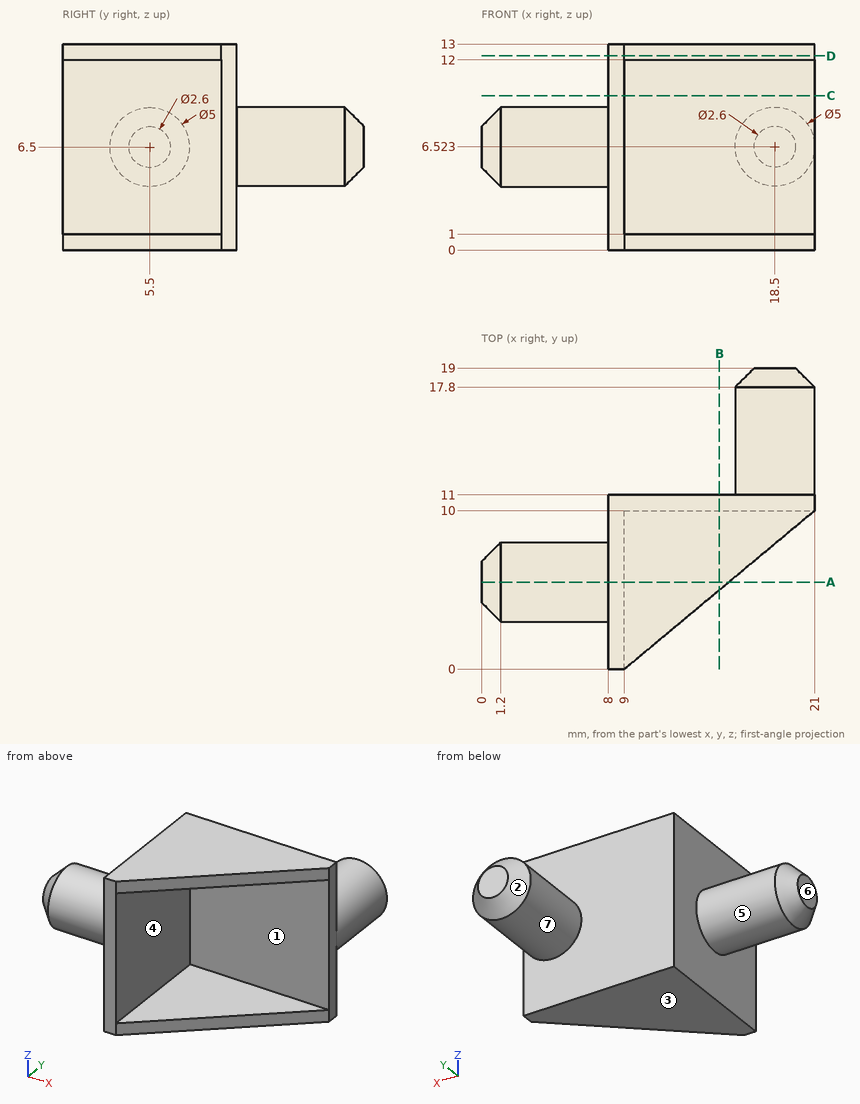
Drawing for the job (mm, zero at the part's lowest x, y, z). A direction names the side the tool comes from. Round coordinates to 2 decimals unless told otherwise and drop trailing zeros. Write each loop counter-clockwise with the first axis right and the second up, starting at its lowest first coordinate (ties: lowest second). Pieces come first, ordered by that corner, then holes. Notation, with made-up numbers: M 3,-27 L 43,-27 A29 ccw 43,-6 Z; hole C 63,29 d9. An arc over 180 degrees is marked long. Answer as a JSON object with one key per item and string values. Group by question number.
(1) Flat gauge pins, fed straight in: pin 1 (4 mm diameter, centred on x = 15, z = 7, fed in from +Y); pin 2 (1 mm diameter, centred on x = 13.5, z = 3, fed in from -Y); pin 3 (4 mm diameter, centred on x = 3, z = 9, fed in from -Y). Where does each tip first touch, or does it go through?
(2) Cut at A-A (y = 5.5). Give the cut face in (x, z).
(3) Which spindle directions (+Z, -Z, +X, -X, +Y, -Y) get a long thin tool onto all of the face, cutting with end or side? Do the marked faces 4, 5, 6 and 7. Say none if no direction does.
(4) Cut at D-D (z = 12.25). Give the cut face in (x, y), and give its area (3 significant figures).
(5) Cut at B-B (x = 15). Give the cut face in (y, z).
(6) Drill centre lines: L1, parallel to Z at x = 10.75, y = 2; L2, parallel to X at y = 10.5, z = 8.75; L3, parallel to Y at x = 13, z = 2. Where is each one in solid material? Low to high.
(7) Cut at C-C (z = 9.75). Give the cut face in (x, y).
(8) Mould opens along Z. For the marked faces 1, 2 and 3 say: pulls with the +Z half, pulls with the -Z half, needs draft (parallel to the pull), parting line crosses it, or undercut.
Responses:
{
 "1": {"pin 1": "stops at y = 18.77", "pin 2": "stops at y = 10", "pin 3": "stops at y = 3.05"},
 "2": {"outline": "M 0,5.2 L 1.2,4 L 8,4 L 8,0 L 15.6,0 L 15.6,1 L 9,1 L 9,12 L 15.6,12 L 15.6,13 L 8,13 L 8,9 L 1.2,9 L 0,7.8 Z"},
 "3": {"face 4": "+X, -Y", "face 5": "-X", "face 6": "+Z, -Z, -X, +Y, -Y", "face 7": "+Y"},
 "4": {"outline": "M 8,0 L 9,0 L 21,10 L 21,11 L 8,11 Z", "area": "83.0 mm2"},
 "5": {"outline": "M 5,0 L 11,0 L 11,13 L 5,13 L 5,12 L 10,12 L 10,1 L 5,1 Z"},
 "6": {"L1": "z = 0 to 1, 12 to 13", "L2": "x = 8 to 21", "L3": "y = 10 to 11"},
 "7": {"outline": "M 8,0 L 9,0 L 9,10 L 21,10 L 21,11 L 8,11 Z"},
 "8": {"face 1": "undercut", "face 2": "parting line crosses it", "face 3": "pulls with the -Z half"}
}
